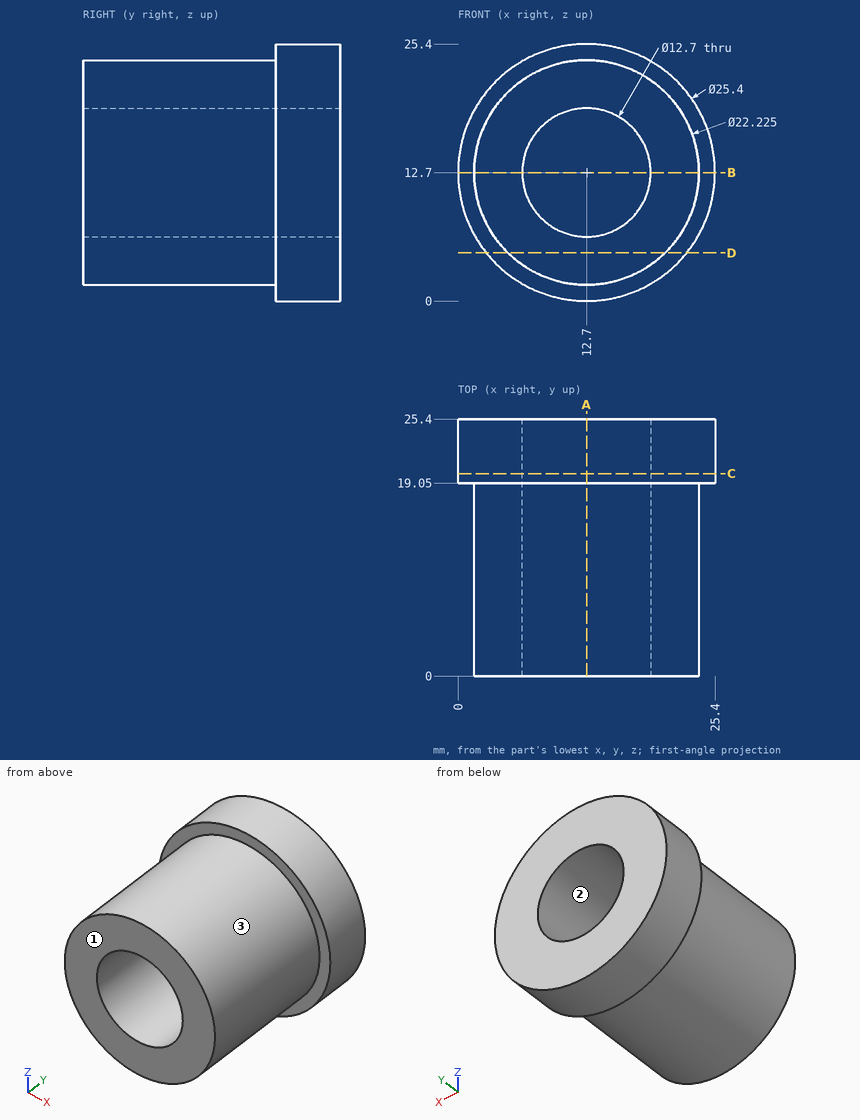
Here's the drawing with two shaded views (mm, measured from the low corner). I have some questions. Give positions to 0.01 mm unless a question says otherwise; leave off trailing zeros. Order: outer loops, then holes, each group sorted by start corner. A loop starts at its lowest first (then second) coordinate and runs counter-clockwise, first axis right, second up.
Q1. We'd pull the mould along X, two halves only. Please class the marked faces 1, 2 and 3: +X half, -X half, draft (parallel to the pull), parting line (faces both ways), or undercut.
Q2. If I drill on line 1 along Z through (x, y) = (12.7, 8.75); line 2 along X through (y, z) = (17.5, 9); line 3 along Z through (x, y) = (14.75, 17.25), over which ranges is the centre line in solid material (lowest first)?
Q3. Suppose I cut it at A-A, the plane x = 12.7. Write out the boundary of the cut face in (y, z), and give its area (3 significant figures).
Q4. Suppose I cut it at B-B, the plane z = 12.7. Write out the boundary of the cut face in (x, y).
Q5. Suppose I cut it at D-D, the plane z = 4.75. Write out the boundary of the cut face in (x, y).
Q6. I'm going to push flat-ended pins straight in: P1, Ø1, axis at y = 18.5, z = 3, coming from the +X side; P2, Ø11.5, axis at x = 12.7, z = 12.7, coming from the +Y side; P3, Ø12.5, axis at x = 9.5, z = 18, coming from the -Y side; P4, Ø5, axis at y = 7, z = 21, coming from the -X side. Where does each tip first touch, or does it pass through?
Q7. Suppose I cut it at C-C, the plane y = 20. Write out the boundary of the cut face in (x, z), and give its area (3 significant figures).
Solution:
1. face 1: draft
1. face 2: undercut
1. face 3: parting line
2. line 1: z = 1.59 to 6.35, 19.05 to 23.81
2. line 2: x = 2.22 to 7.54, 17.86 to 23.18
2. line 3: z = 1.78 to 6.69, 18.71 to 23.62
3. outline: (0, 1.59) - (19.05, 1.59) - (19.05, 0) - (25.4, 0) - (25.4, 6.35) - (0, 6.35) - close; (0, 19.05) - (25.4, 19.05) - (25.4, 25.4) - (19.05, 25.4) - (19.05, 23.81) - (0, 23.81) - close
3. area: 262 mm2
4. outline: (0, 19.05) - (1.59, 19.05) - (1.59, 0) - (6.35, 0) - (6.35, 25.4) - (0, 25.4) - close; (19.05, 0) - (23.81, 0) - (23.81, 19.05) - (25.4, 19.05) - (25.4, 25.4) - (19.05, 25.4) - close
5. outline: (2.8, 19.05) - (4.94, 19.05) - (4.94, 0) - (20.46, 0) - (20.46, 19.05) - (22.6, 19.05) - (22.6, 25.4) - (2.8, 25.4) - close
6. P1: stops at x = 18.93
6. P2: passes through
6. P3: stops at y = 0
6. P4: stops at x = 3.22
7. outline: circle Ø25.4 at (12.7, 12.7); hole circle Ø12.7 at (12.7, 12.7)
7. area: 380 mm2
